from build123d import *

# Parameters (mm, degrees)
SKIZZE1_R                       = 14
AUFSATZ_LINEAR_AUSTRAGEN1_DEPTH = 4
SKIZZE3_R                       = 2.1
SCHNITT_LINEAR_AUSTRAGEN1_DEPTH = 5
SKIZZE2_R                       = 10.5
AUFSATZ_LINEAR_AUSTRAGEN2_DEPTH = 8
SCHNITT_LINEAR_AUSTRAGEN2_REACH = 10
SKIZZE5_R                       = 3
SKIZZE6_R                       = 2.5
SCHNITT_LINEAR_AUSTRAGEN3_DEPTH = 13
SCHNITT_LINEAR_AUSTRAGEN4_REACH = 26.5
SKIZZE7_R                       = 1.25


with BuildPart() as part:
    # Skizze1 → Aufsatz-Linear austragen1 (new body)
    with BuildSketch(Plane.XY):
        Circle(SKIZZE1_R)
    extrude(amount=AUFSATZ_LINEAR_AUSTRAGEN1_DEPTH)

    # Skizze3 → Schnitt-Linear austragen1 (cut, through all)
    with BuildSketch(Plane.XY.offset(4)):
        with Locations((-8, 4.618802154)):
            Circle(SKIZZE3_R)
        with Locations((8, 4.618802154)):
            Circle(SKIZZE3_R)
        with Locations((0, -9.237604307)):
            Circle(SKIZZE3_R)
    extrude(amount=-SCHNITT_LINEAR_AUSTRAGEN1_DEPTH, mode=Mode.SUBTRACT)

    # Skizze2 → Aufsatz-Linear austragen2 (add)
    with BuildSketch(Plane.XY.offset(4)):
        Circle(SKIZZE2_R)
    extrude(amount=AUFSATZ_LINEAR_AUSTRAGEN2_DEPTH)

    # Skizze5 → Schnitt-Linear austragen2 (cut, up to next)
    with BuildSketch(Plane(origin=(0, 0, 4), x_dir=(-1, 0, 0), z_dir=(0, 0, -1)), mode=Mode.PRIVATE) as schnitt_linear_austragen2_sk1:
        with Locations((-8, 4.618802154)):
            Circle(SKIZZE5_R)
    schnitt_linear_austragen2_tool1 = extrude(schnitt_linear_austragen2_sk1.sketch, amount=-SCHNITT_LINEAR_AUSTRAGEN2_REACH, mode=Mode.PRIVATE) & part.part
    add(schnitt_linear_austragen2_tool1.solids().sort_by_distance((8, 4.618802, 4))[0], mode=Mode.SUBTRACT)
    # Skizze5 → Schnitt-Linear austragen2 (cut, up to next)
    with BuildSketch(Plane(origin=(0, 0, 4), x_dir=(-1, 0, 0), z_dir=(0, 0, -1)), mode=Mode.PRIVATE) as schnitt_linear_austragen2_sk2:
        with Locations((8, 4.618802154)):
            Circle(SKIZZE5_R)
    schnitt_linear_austragen2_tool2 = extrude(schnitt_linear_austragen2_sk2.sketch, amount=-SCHNITT_LINEAR_AUSTRAGEN2_REACH, mode=Mode.PRIVATE) & part.part
    add(schnitt_linear_austragen2_tool2.solids().sort_by_distance((-8, 4.618802, 4))[0], mode=Mode.SUBTRACT)
    # Skizze5 → Schnitt-Linear austragen2 (cut, up to next)
    with BuildSketch(Plane(origin=(0, 0, 4), x_dir=(-1, 0, 0), z_dir=(0, 0, -1)), mode=Mode.PRIVATE) as schnitt_linear_austragen2_sk3:
        with Locations((0, -9.237604307)):
            Circle(SKIZZE5_R)
    schnitt_linear_austragen2_tool3 = extrude(schnitt_linear_austragen2_sk3.sketch, amount=-SCHNITT_LINEAR_AUSTRAGEN2_REACH, mode=Mode.PRIVATE) & part.part
    add(schnitt_linear_austragen2_tool3.solids().sort_by_distance((0, -9.237604, 4))[0], mode=Mode.SUBTRACT)

    # Skizze6 → Schnitt-Linear austragen3 (cut, through all)
    with BuildSketch(Plane.XY.offset(12)):
        Circle(SKIZZE6_R)
    extrude(amount=-SCHNITT_LINEAR_AUSTRAGEN3_DEPTH, mode=Mode.SUBTRACT)

    # Skizze7 → Schnitt-Linear austragen4 (cut, up to next)
    with BuildSketch(Plane(origin=(0, 10.5, 0), x_dir=(1, 0, 0), z_dir=(0, 1, 0)), mode=Mode.PRIVATE) as schnitt_linear_austragen4_sk1:
        with Locations((0, -8)):
            Circle(SKIZZE7_R)
    schnitt_linear_austragen4_tool1 = extrude(schnitt_linear_austragen4_sk1.sketch, amount=-SCHNITT_LINEAR_AUSTRAGEN4_REACH, mode=Mode.PRIVATE) & part.part
    add(schnitt_linear_austragen4_tool1.solids().sort_by_distance((0, 10.5, 8))[0], mode=Mode.SUBTRACT)


solid = part.part
The listing builds one solid part. Answer for the finished solid, in the listing's coordinates (mm). A direction names the side the tool comes from. Round coordinates to 2 decimals unless told otherwise and drop trailing zeros. Write each loop counter-clockwise with the first axis right and the second up, starting at its lowest first coordinate (ties: lowest second). Pieces come first, ordered by that corner, then holes. Notation, with made-up numbers: M 18,30.5 L 33,30.5 A24 cw 33,50.5 Z; hole C 10.5,84.25 d2. An arc over 180 degrees is marked long. Write each question's results on one line, items separated by ' | '. Start each with the question number.
(1) Each of these flat-tipped pins is pushed along its axis until it touches: P1, Ø3, axis at x = 0, z = 8, coming from the -Y side; P2, Ø3, axis at x = 11, y = 6, coming from the +Z side; P3, Ø2, axis at x = -2, z = 4, coming from the -Y side. Where does it stop, or does it pass through?
(2) The part is cut by section D-D, the plane x = -3.75. Write down the section's boundary in (y, z).
(3) The part is cut by section B-B, the plane z = 6. Write down the section's boundary in (x, y).
(4) Find the intervals of material crossed by line 1 (Y direction, x = 0, z = 3.2); line 2 (X direction, y = -8.5, z = 9.5); line 3 (X direction, y = -0.25, z = 10.75), in increasing order.
(5) The part is cut by section C-C, the plane x = 9.25. Write down the section's boundary in (y, z).
(6) The part is cut by section A-A, the plane y = 0. Write down the section's boundary in (x, z), and give its area (3 significant figures).
(7) Determine the mould class of faces 1 (the cylindrical face through (9.036, -5.348, 7.944)), 2 (the flat face through (3, 0, 0)), 3 (the cylindrical face through (5.442, 3.052, 7.944)), 4 (the cylindrical face through (1.899, 10.327, 7.944)) for opening direction X: +X half, -X half, draft (parallel to the pull), parting line (faces both ways), or undercut.
(8) For faces 5 (the cylindrical face through (-0.27, 6.39, 9.22)), 6 (the flat face through (0, 3, 12)), 7 (the cylindrical face through (6.334, 3.341, 2.028)), 8 (the cylindrical face through (-5.36, 3.19, 7.94)), 9 (the cylindrical face through (-9.15, -5.15, 7.94)), determine the directions among +Z, -Z, +X, -X, +Y, -Y from which every point of the face is accessible in a straight line to the end or side of a thin tool.
Worked answers:
1) P1: stops at y = -6.64 | P2: stops at z = 4 | P3: stops at y = -13.96
2) outline: M -13.49,0 L 13.49,0 L 13.49,4 L 9.81,4 L 9.81,12 L -9.81,12 L -9.81,4 L -13.49,4 Z
3) outline: M -10.18,2.56 A10.5 ccw -2.87,-10.1 A3 cw long 2.87,-10.1 A10.5 ccw 10.18,2.56 A3 cw long 7.31,7.54 A10.5 ccw -7.31,7.54 A3 cw long Z; hole C 0,0 d5
4) line 1: y = -14 to -11.34, -7.14 to -2.5, 2.5 to 14 | line 2: x = -6.16 to -2.91, 2.91 to 6.16 | line 3: x = -10.5 to -2.49, 2.49 to 10.5
5) outline: M -10.51,0 L 2.93,0 L 2.93,4 L 1.89,4 L 1.89,12 L -4.97,12 L -4.97,4 L -10.51,4 Z; M 6.31,0 L 10.51,0 L 10.51,4 L 6.31,4 Z
6) outline: M -14,0 L -2.5,0 L -2.5,12 L -10.5,12 L -10.5,4 L -14,4 Z; M 2.5,0 L 14,0 L 14,4 L 10.5,4 L 10.5,12 L 2.5,12 Z | area: 220 mm²
7) face 1: +X half | face 2: draft | face 3: undercut | face 4: parting line
8) face 5: +Y | face 6: +Z, +X, -X, +Y, -Y | face 7: +Z, -Z | face 8: +Z | face 9: +Z, -X
